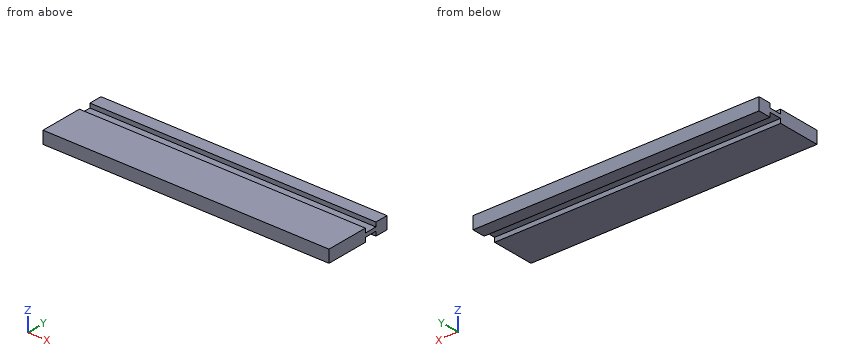
from build123d import *

# Parameters (mm, degrees)
CROQUIS1_W              = 460
CROQUIS1_H              = 110
SALIENTE_EXTRUIR1_DEPTH = 20
CROQUIS8_W              = 480
CROQUIS8_H              = 20
CORTAR_EXTRUIR3_DEPTH   = 7
CROQUIS9_W              = 470
CROQUIS9_H              = 20
CORTAR_EXTRUIR4_DEPTH   = 7


with BuildPart() as part:
    # Croquis1 → Saliente-Extruir1 (new body)
    with BuildSketch(Plane.XY):
        Rectangle(CROQUIS1_W, CROQUIS1_H)
    extrude(amount=SALIENTE_EXTRUIR1_DEPTH)

    # Croquis8 → Cortar-Extruir3 (cut)
    with BuildSketch(Plane.XY.offset(20)):
        with Locations((-10, 24)):
            Rectangle(CROQUIS8_W, CROQUIS8_H)
    extrude(amount=-CORTAR_EXTRUIR3_DEPTH, mode=Mode.SUBTRACT)

    # Croquis9 → Cortar-Extruir4 (cut)
    with BuildSketch(Plane(origin=(0, 0, 0), x_dir=(-1, 0, 0), z_dir=(0, 0, -1))):
        with Locations((-5, 24)):
            Rectangle(CROQUIS9_W, CROQUIS9_H)
    extrude(amount=-CORTAR_EXTRUIR4_DEPTH, mode=Mode.SUBTRACT)


solid = part.part
Source: CAD feature listing. Evaluate the final solid. Frame: model axes, mm. Give positions to 0.01 mm unless a question says otherwise; leave off trailing zeros. Write each loop counter-clockwise with the first axis right and the second up, starting at its lowest first coordinate (ties: lowest second). Pieces come first, ordered by that corner, then holes. Notation, with made-up numbers: (-16, 70.5) - (22, 70.5) arc R8 ccw to (22, 78.5) - close; hole circle Ø5 at (21.5, 73). An arc over 180 degrees is marked (long way). Write item = value, one per line. Start each with the question number.
Q1. Cut plane A-A, the plane z = 16.5. Return loops of the section in (x, y).
Q2. Cut plane B-B, the plane x = -172. Return loops of the section in (y, z), then the cut area to 3 significant figures.
Q3. Cut plane C-C, the plane y = 30. Return loops of the section in (x, z).
Q4. Material intervals for probe 1 along Y at (x, z) = (45, 15.5); probe 2 along Z at (x, y) = (-73, 17.5), sorted ascending.
Computed values:
q1.outline = (-230, -55) - (230, -55) - (230, 14) - (-230, 14) - close; (-230, 34) - (230, 34) - (230, 55) - (-230, 55) - close
q2.outline = (-55, 0) - (14, 0) - (14, 7) - (34, 7) - (34, 0) - (55, 0) - (55, 20) - (34, 20) - (34, 13) - (14, 13) - (14, 20) - (-55, 20) - close
q2.area = 1,920 mm²
q3.outline = (-230, 7) - (230, 7) - (230, 13) - (-230, 13) - close
q4.probe_1 = -55 to 14, 34 to 55
q4.probe_2 = 7 to 13
